Model file for the job. Use its own axes, mm. A direction names the side the tool comes from. Coordinates: 2 decimals unless noted, no trailing zeros. Write each loop counter-clockwise with the first axis right and the second up, starting at its lowest first coordinate (ties: lowest second). Pieces come first, ordered by that corner, then holes. Notation, with made-up numbers: M -20.5,43 L 1.5,43 A3 ccw 1.5,47 Z; hole C 86.5,-19 d7. An arc over 180 degrees is marked long. One line per question, with ' | ' between items. Start each with the question number.
(1) Cut at A-A (y = 0). Write the cut outline in (x, z).
(2) Wall check: probe 1 along Y at (x, z) = (0, 1.2); probe 2 along X at (y, z) = (28.5, 3.35); probe 3 along Y at (x, z) = (-20, 2.65). Give the ranges that are in metal, low to high.
(3) Cut at C-C (z = 4.5). Write the cut outline in (x, y), plus the area to 3 significant figures.
(4) Cut at B-B (x = 0). Write the cut outline in (y, z), plus the area to 3 significant figures.
(5) Tool access for faces 4 (the face through (-34, -10, 5.5)), 5 (the face through (-43, 2.75, 3)): list every direction of +Z, -Z, +X, -X, +Y, -Y with a clear straight run to the whole face (end or side of a thin tool).
(6) Cut at D-D (y = 14). Write the cut outline in (x, z).
(7) Flat gauge pins, fed straight in: pin 1 Ø1.6 at (x, z) = (43, 3) entering from -Y; pin 2 Ø1.6 at (x, z) = (43, 3.5) entering from +Y. Where does each tip first touch, or does it go through?
(8) Two-plate mould, pull along X, no slides. Class faces 1 (the face through (47.69, -15.02, 2.71)), 2 (the face through (42, 2.75, 3)), 3 (the face through (-34, -10, 0)): +X half, -X half, draft (parallel to the pull), parting line (faces both ways), or undercut.
Autodesk Inventor part; units mm, degrees
ref_plane "YZ Plane" through (0, 0, 0) normal (1, 0, 0) x (0, 1, 0)
ref_plane "XZ Plane" through (0, 0, 0) normal (0, 1, 0) x (-1, 0, 0)
ref_plane "XY Plane" through (0, 0, 0) normal (0, 0, 1) x (1, 0, 0)
sketch "Sketch1" plane through (0, 0, 0) normal (0, 0, 1) x (1, 0, 0)
  circle A0 centre (0, 0) radius 50
  circle A1 centre (0, 0) radius 35
  dimension "d0" = 100
  dimension "d1" = 70
extrude "Extrusion1" add sketch "Sketch1" along normal blind 5.5
sketch "Sketch4" plane through (0, 0, 5.5) normal (0, 0, 1) x (1, 0, 0)
  line L0 (39.75, 2.75) -> (45.25, 2.75)
  line L1 (45.25, 2.75) -> (45.25, -2.75)
  line L2 (45.25, -2.75) -> (39.75, -2.75)
  line L3 (39.75, -2.75) -> (39.75, 2.75)
  line L4 (-39.75, -2.75) -> (-45.25, -2.75)
  line L5 (-45.25, -2.75) -> (-45.25, 2.75)
  line L6 (-45.25, 2.75) -> (-39.75, 2.75)
  line L7 (-39.75, 2.75) -> (-39.75, -2.75)
  point P0 (0, 0)
  dimension "d13" = 5.5
  dimension "d14" = 5.5
  dimension "d17" = 360
extrude "Extrusion3" cut sketch "Sketch4" against normal blind 10
properties part number "central"
Filled in:
1) outline: M -50,0 L -45.25,0 L -45.25,5.5 L -50,5.5 Z; M -39.75,0 L -35,0 L -35,5.5 L -39.75,5.5 Z; M 35,0 L 39.75,0 L 39.75,5.5 L 35,5.5 Z; M 45.25,0 L 50,0 L 50,5.5 L 45.25,5.5 Z
2) probe 1: -50 to -35, 35 to 50 | probe 2: -41.08 to -20.32, 20.32 to 41.08 | probe 3: -45.83 to -28.72, 28.72 to 45.83
3) outline: C 0,0 d100; hole M -45.25,-2.75 L -39.75,-2.75 L -39.75,2.75 L -45.25,2.75 Z; hole C 0,0 d70; hole M 39.75,-2.75 L 45.25,-2.75 L 45.25,2.75 L 39.75,2.75 Z | area: 3,950 mm²
4) outline: M -50,0 L -35,0 L -35,5.5 L -50,5.5 Z; M 35,0 L 50,0 L 50,5.5 L 35,5.5 Z | area: 165 mm²
5) face 4: +Z, +X, -X, +Y, -Y | face 5: +Z, -Z
6) outline: M -48,0 L -32.08,0 L -32.08,5.5 L -48,5.5 Z; M 32.08,0 L 48,0 L 48,5.5 L 32.08,5.5 Z
7) pin 1: y = -26.82 | pin 2: y = 26.82
8) face 1: parting line | face 2: undercut | face 3: draft
